Model file for the job. Use its own axes, mm. Face numbers are marked on the shaded views. A direction names the side the tool comes from. Give positions to 0.01 mm unless a question says otherwise; leave off trailing zeros. Order: outer loops, then holes, each group sorted by start corner. A loop starts at its lowest first (then second) coordinate and runs counter-clockwise, first axis right, second up. Notation, with made-up numbers: (8, 38) - (12, 38) arc R19 cw to (12, 53) - close; hole circle Ø2 at (45, -2). An arc over 180 degrees is marked (long way). Use CSV: the item, a comma, the result in double quotes. Start each with the question number.
(1) Band-saw the part on C-C, the plane z = -5.75. Give the cut face in (x, y).
(2) Band-saw the part on B-B, the plane x = -1.25. Give the cut face in (y, z), then the cut area to 3 significant figures.
(3) Band-saw the part on A-A, the plane y = 0. Give the cut face in (x, z), then the cut area to 3 significant figures.
(4) Band-saw the part on D-D, the plane z = 5.5. Give the cut face in (x, y), then the cut area to 3 significant figures.
(5) Probe L1, parallel to Z at x = 1.75, y = 4.25; L2, parallel to Y at x = -2.5, z = -3; L3, parallel to Y at x = 0.25, z = 4. List the from-to ranges inside material, lowest first.
(6) Drop flat-ended pins along their axis: pin 1 Ø1 at (x, z) = (2.5, -2.5) entering from -Y; pin 2 Ø3 at (y, z) = (2.5, -8) entering from +X; pin 3 Ø6 at (y, z) = (1.5, -6.5) entering from +X. Give the stop position or say it passes through.
(7) Tool access for the marked faces 1, 2 and 3: list every direction of +Z, -Z, +X, -X, +Y, -Y with a clear straight run to the whole face (end or side of a thin tool).
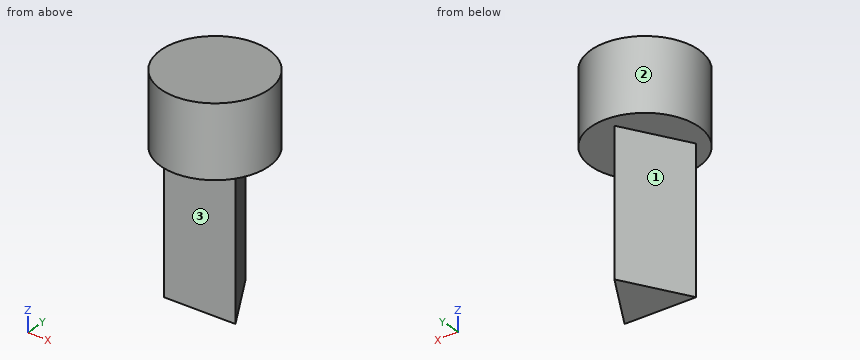
Autodesk Inventor part; units mm, degrees
ref_plane "YZ Plane" through (0, 0, 0) normal (1, 0, 0) x (0, 1, 0)
ref_plane "XZ Plane" through (0, 0, 0) normal (0, 1, 0) x (-1, 0, 0)
ref_plane "XY Plane" through (0, 0, 0) normal (0, 0, 1) x (1, 0, 0)
sketch "Sketch1" plane through (0, 0, 0) normal (0, 0, 1) x (1, 0, 0)
  line L0 (0, 10.9985) -> (9.525, -5.4993)
  line L1 (9.525, -5.4993) -> (-9.525, -5.4993)
  line L2 (-9.525, -5.4993) -> (0, 10.9985)
  line L3 (-4.2333, -2.4441) -> (0, 4.8882)
  line L4 (0, 4.8882) -> (4.2333, -2.4441)
  line L5 (4.2333, -2.4441) -> (-4.2333, -2.4441)
  point P0 (0, 0)
  point P1 (0, 0)
  point P2 (0, 0)
  dimension "d0" = 19.05
  dimension "d1" = 8.4667
extrude "Extrusion1" add sketch "Sketch1" against normal blind 16.9333 contours L3 L4 L5
sketch "Sketch2" plane through (0, 0, 0) normal (0, 0, 1) x (1, 0, 0)
  circle A0 centre (0, 0) radius 6.35
  dimension "d4" = 12.7
extrude "Extrusion2" add sketch "Sketch2" along normal blind 8.4667
properties part number "Driver Shaft" material "ABS Plastic"
Answer block:
1,outline,"(-4.23, -2.44) - (4.23, -2.44) - (0, 4.89) - close"
2,outline,"(-6.23, 0) - (-2.44, 0) - (-2.44, -16.93) - (2.72, -16.93) - (2.72, 0) - (6.23, 0) - (6.23, 8.47) - (-6.23, 8.47) - close"
2,area,"193 mm2"
3,outline,"(-6.35, 0) - (-2.82, 0) - (-2.82, -16.93) - (2.82, -16.93) - (2.82, 0) - (6.35, 0) - (6.35, 8.47) - (-6.35, 8.47) - close"
3,area,"203 mm2"
4,outline,"circle Ø12.7 at (0, 0)"
4,area,"127 mm2"
5,L1,"z = 0 to 8.47"
5,L2,"y = -2.44 to 0.56"
5,L3,"y = -6.35 to 6.35"
6,pin 1,"stops at y = -2.44"
6,pin 2,"stops at x = 2.24"
6,pin 3,"stops at x = 3.69"
7,face 1,"-Z, -X, +Y"
7,face 2,"+Z, -Z"
7,face 3,"-Z, +X, -X, -Y"
